Part model, mm, in its own coordinate system. A direction names the side the tool comes from. Round coordinates to 2 decimals unless told otherwise and drop trailing zeros. Loops run counter-clockwise (first coordinate to the right, second up) from the corner with the lowest first, then second, coordinate; pieces in that order, holes last. Notation, with made-up numbers: (48.25, 47) -> (60.25, 47) arc R10 cw to (60.25, 60) -> close; hole circle Ø3 at (26.25, 65). An arc over 180 degrees is marked (long way). Use a Markdown table: item, result. Add a question column.
Item 1: Cut at B-B, the plane y = 4. List the corners of the cut face in (x, z).
Item 2: Probe line 1 (Z direction, x = -0.5, y = -4); line 2 (Z direction, x = 3.5, y = -4.5); line 3 (X direction, y = -2.5, z = -2). List the from-to ranges inside material, lowest first. Write a range as [from, to].
Item 3: Which spindle directions (+Z, -Z, +X, -X, +Y, -Y) get a long thin tool onto all of the face, cutting with end or side? Do faces 1 (the face through (0.7, 2.3, -27.1)), 2 (the face through (0, -9.525, -16)). Say none if no direction does.
Item 4: Cut at A-A, the plane x = 0. List the corners of the cut face in (y, z) (1 decimal).
Item 5: Flat gauge pins, fed straight in: pin 1 (1.5 mm diameter, centred on x = -1.5, z = -9, fed in from -Y); pin 2 (2 mm diameter, centred on y = 1.5, z = -29, fed in from -X); pin 3 (2 mm diameter, centred on x = -0.5, y = -3.5, fed in from -Z). Where does each tip first touch, or does it go through?
Autodesk Inventor part; units mm, degrees
ref_plane "YZ Plane" through (0, 0, 0) normal (1, 0, 0) x (0, 1, 0)
ref_plane "XZ Plane" through (0, 0, 0) normal (0, 1, 0) x (-1, 0, 0)
ref_plane "XY Plane" through (0, 0, 0) normal (0, 0, 1) x (1, 0, 0)
sketch "Sketch1" plane through (0, 0, 0) normal (1, 0, 0) x (0, 1, 0)
  line L0 (-9.525, 36.5125) -> (9.525, 36.5125)
  line L1 (9.525, 36.5125) -> (9.525, -36.5125)
  line L2 (9.525, -36.5125) -> (-9.525, -36.5125)
  line L3 (-9.525, -36.5125) -> (-9.525, 36.5125)
  line L4 (-9.525, 36.5125) -> (9.525, -36.5125) construction
  line L5 (9.525, 36.5125) -> (-9.525, -36.5125) construction
  point P0 (0, 0)
  dimension "d0" = 19.05
  dimension "d1" = 73.025
extrude "Extrusion1" add sketch "Sketch1" along normal mid plane 9.525
sketch "Sketch2" plane through (4.7625, 0, 0) normal (1, 0, 0) x (0, 0, -1)
  line L0 (-36.5125, 9.525) -> (-36.5125, -9.525)
  line L1 (-36.5125, 9.525) -> (14.2875, 9.525)
  line L2 (14.2875, 9.525) -> (14.2875, -1.5875)
  line L3 (14.2875, -1.5875) -> (-36.5125, -1.5875)
  line L4 (-36.5125, -1.5875) -> (-36.5125, 9.525)
  line L5 (-36.5125, -9.525) -> (36.5125, -9.525)
  point P0 (0, 0)
  dimension "d4" = 50.8
  dimension "d6" = 7.9375
extrude "Extrusion2" cut sketch "Sketch2" against normal blind 9.525
sketch "Sketch3" plane through (4.7625, 0, 0) normal (1, 0, 0) x (0, 0, -1)
  line L0 (36.5125, -9.525) -> (-36.5125, -9.525)
  line L1 (36.5125, -9.525) -> (17.4625, -9.525)
  line L2 (17.4625, -9.525) -> (17.4625, 1.5875)
  line L3 (17.4625, 1.5875) -> (36.5125, 1.5875)
  line L4 (36.5125, 1.5875) -> (36.5125, -9.525)
  line L5 (14.2875, 9.525) -> (14.2875, -1.5875)
  line L6 (36.5125, 9.525) -> (14.2875, 9.525)
  point P0 (0, 0)
  dimension "d9" = 3.175
  dimension "d10" = 7.9375
extrude "Extrusion3" cut sketch "Sketch3" against normal blind 9.525
sketch "Sketch4" plane through (4.7625, 0, 0) normal (1, 0, 0) x (0, 0, -1)
  line L0 (-36.5125, -1.5875) -> (-36.5125, -9.525)
  line L1 (-36.5125, -9.525) -> (14.2875, -9.525)
  line L2 (14.2875, -9.525) -> (14.2875, -7.9375)
  line L3 (14.2875, -7.9375) -> (-36.5125, -7.9375)
  line L4 (-36.5125, -7.9375) -> (-36.5125, -9.525)
  point P0 (0, 0)
  dimension "d13" = 50.8
  dimension "d14" = 1.5875
extrude "Extrusion4" cut sketch "Sketch4" against normal blind 9.525
sketch "Sketch5" plane through (4.7625, 0, 0) normal (1, 0, 0) x (0, 0, -1)
  line L0 (36.5125, 9.525) -> (36.5125, 1.5875)
  line L1 (36.5125, 9.525) -> (17.4625, 9.525)
  line L2 (17.4625, 9.525) -> (17.4625, 7.9375)
  line L3 (17.4625, 7.9375) -> (36.5125, 7.9375)
  line L4 (36.5125, 7.9375) -> (36.5125, 9.525)
  point P0 (0, 0)
  dimension "d17" = 19.05
  dimension "d18" = 1.5875
extrude "Extrusion5" cut sketch "Sketch5" against normal blind 9.525
sketch "Sketch7" plane through (4.7625, 1.5875, -36.5125) normal (0, 0, -1) x (-1, 0, 0)
  line L0 (9.525, 6.35) -> (9.525, 0)
  line L1 (0, 0) -> (0, 6.35)
  line L2 (9.525, 6.35) -> (0, 6.35)
  line L3 (0, 6.35) -> (0, 0)
  line L4 (0, 0) -> (9.525, 0)
  line L5 (9.525, 0) -> (9.525, 6.35)
  circle A0 centre (4.7625, 3.81) radius 3.175
  point P0 (4.7625, -1.5875)
  dimension "d26" = 6.35
  dimension "d27" = 4.7625
  dimension "d28" = 3.81
extrude "Extrusion7" add sketch "Sketch7" against normal blind 19.05 contours A0 L2 | L2 A0
sketch "Sketch6" plane through (-4.7625, -1.5875, 36.5125) normal (0, 0, 1) x (1, 0, 0)
  line L0 (9.525, -6.35) -> (0, -6.35)
  line L1 (9.525, 0) -> (0, 0)
  line L2 (0, -6.35) -> (9.525, -6.35)
  line L3 (9.525, -6.35) -> (9.525, 0)
  line L4 (9.525, 0) -> (0, 0)
  line L5 (0, 0) -> (0, -6.35)
  circle A0 centre (4.7625, -3.6322) radius 3.175
  point P0 (4.7625, 1.5875)
  dimension "d21" = 6.35
  dimension "d22" = 3.6322
  dimension "d23" = 4.7625
extrude "Extrusion6" add sketch "Sketch6" against normal blind 50.8
fillet "Fillet1" radius 1.5875 4 edges at (4.7625, 9.525, -15.875) (-4.7625, 9.525, -15.875) (4.7625, -9.525, -15.875) (-4.7625, -9.525, -15.875)
sketch "Sketch8" plane through (4.7625, 1.5875, -36.5125) normal (0, 0, -1) x (-1, 0, 0)
  arc A0 (6.6675, 6.35) -> (2.8575, 6.35) centre (4.7625, 3.81) ccw
  circle A1 centre (4.7625, 3.81) radius 3.175
  line L0 (0, 6.35) -> (2.8575, 6.35)
  line L1 (2.8575, 6.35) -> (0, 6.35)
  line L2 (0, 0) -> (0, 6.35)
  line L3 (0, 0) -> (9.525, 0)
  line L4 (9.525, 6.35) -> (9.525, 0)
  line L5 (2.8575, 6.35) -> (0, 6.35)
  line L6 (0, 0) -> (0, 6.35)
  line L7 (0, 0) -> (9.525, 0)
  line L8 (9.525, 6.35) -> (9.525, 0)
  line L9 (9.525, 6.35) -> (6.6675, 6.35)
  arc A2 (6.6675, 6.35) -> (2.8575, 6.35) centre (4.7625, 3.81) ccw
  line L10 (0, 0) -> (9.525, 0)
  line L11 (0, 6.35) -> (0, 0)
  line L12 (0, 0) -> (9.525, 0)
  line L13 (9.525, 0) -> (9.525, 6.35)
  point P0 (4.7625, -1.5875)
extrude "Extrusion8" cut sketch "Sketch8" against normal blind 19.05 contours L9 L4 L3 L2 L0 A1
sketch "Sketch9" plane through (-4.7625, -1.5875, 36.5125) normal (0, 0, 1) x (1, 0, 0)
  arc A0 (3.1211, -6.35) -> (6.4039, -6.35) centre (4.7625, -3.6322) ccw
  line L0 (0, -6.35) -> (3.1211, -6.35)
  arc A1 (3.1211, -6.35) -> (6.4039, -6.35) centre (4.7625, -3.6322) ccw
  line L1 (6.4039, -6.35) -> (9.525, -6.35)
  line L2 (9.525, 0) -> (9.525, -6.35)
  line L3 (9.525, 0) -> (0, 0)
  line L4 (0, -6.35) -> (0, 0)
  arc A2 (6.4039, -6.35) -> (3.1211, -6.35) centre (4.7625, -3.6322) ccw
  arc A3 (3.1211, -6.35) -> (6.4039, -6.35) centre (4.7625, -3.6322) ccw
  line L5 (0, -6.35) -> (0, 0)
  line L6 (3.1211, -6.35) -> (0, -6.35)
  line L7 (0, -6.35) -> (0, 0)
  line L8 (9.525, 0) -> (0, 0)
  line L9 (0, 0) -> (9.525, 0)
  line L10 (9.525, 0) -> (9.525, -6.35)
  line L11 (9.525, 0) -> (9.525, -6.35)
  line L12 (9.525, -6.35) -> (6.4039, -6.35)
  line L13 (9.525, -6.35) -> (6.4039, -6.35)
  point P0 (4.7625, 1.5875)
extrude "Extrusion9" cut sketch "Sketch9" against normal blind 50.8 contours L0 L4 L3 L2 L1 A2
properties part number "CrankShaft"
A:
| question | item | result |
|---|---|---|
| 1 | outline | (-4.76, -17.46) -> (-2.85, -17.46) -> (-2.85, -36.51) -> (2.85, -36.51) -> (2.85, -17.46) -> (4.76, -17.46) -> (4.76, -14.29) -> (-4.76, -14.29) -> close |
| 2 | line 1 | z = [-17.46, 36.51] |
| 2 | line 2 | z = [-17.46, -14.29] |
| 2 | line 3 | x = [-1.64, 1.64] |
| 3 | face 1 | -Z |
| 3 | face 2 | +Z, -Z, +X, -X, -Y |
| 4 | outline | (-9.5, -17.5) -> (2.2, -17.5) -> (2.2, -36.5) -> (8.6, -36.5) -> (8.6, -17.5) -> (9.5, -17.5) -> (9.5, -14.3) -> (-2, -14.3) -> (-2, 36.5) -> (-8.4, 36.5) -> (-8.4, -14.3) -> (-9.5, -14.3) -> close |
| 5 | pin 1 | stops at y = -8.3 |
| 5 | pin 2 | stops at x = -1.3 |
| 5 | pin 3 | stops at z = -17.46 |
